from build123d import *

# Parameters (mm, degrees)
SKETCH1_R           = 46.355
BOSS_EXTRUDE1_DEPTH = 6.35
SKETCH2_R           = 20.955
BOSS_EXTRUDE2_DEPTH = 50.8
CUT_EXTRUDE1_REACH  = 59.15
SKETCH3_3_R         = 13.0175
CUT_EXTRUDE2_DEPTH  = 34.29
CUT_EXTRUDE3_REACH  = 48.355
SKETCH5_5_R         = 2.2479
CUT_EXTRUDE7_DEPTH  = 9.525
CIRPATTERN1_COUNT   = 4
CUT_EXTRUDE8_REACH  = 95.345
SKETCH6_R           = 2.60985
SKETCH6_4_R         = 4.7625
CUT_EXTRUDE9_DEPTH  = 32.72
CHAMFER1_SIZE       = 1


with BuildPart() as part:
    # Sketch1 → Boss-Extrude1 (new body)
    with BuildSketch(Plane(origin=(0, 0, 0), x_dir=(1, 0, 0), z_dir=(0, 1, 0))):
        Circle(SKETCH1_R)
    extrude(amount=BOSS_EXTRUDE1_DEPTH)

    # Sketch2 → Boss-Extrude2 (add)
    with BuildSketch(Plane(origin=(0, 6.35, 0), x_dir=(1, 0, 0), z_dir=(0, 1, 0))):
        Circle(SKETCH2_R)
    extrude(amount=BOSS_EXTRUDE2_DEPTH)

    # Sketch3 → Cut-Extrude1 (cut, up to next)
    with BuildSketch(Plane(origin=(0, 57.15, 0), x_dir=(1, 0, 0), z_dir=(0, 1, 0)), mode=Mode.PRIVATE) as cut_extrude1_sk1:
        with BuildLine():
            Line((-2.84, -1.921572533), (-2.84, 1.921572533))
            ThreePointArc((-2.84, 1.921572533), (3.429, 0), (-2.84, -1.921572533))
        make_face()
    cut_extrude1_tool1 = extrude(cut_extrude1_sk1.sketch, amount=-CUT_EXTRUDE1_REACH, mode=Mode.PRIVATE) & part.part
    add(cut_extrude1_tool1.solids().sort_by_distance((0.133614, 57.15, 0))[0], mode=Mode.SUBTRACT)

    # Sketch3_3 → Cut-Extrude2 (cut)
    with BuildSketch(Plane(origin=(0, 57.15, 0), x_dir=(1, 0, 0), z_dir=(0, 1, 0))):
        Circle(SKETCH3_3_R)
    extrude(amount=-CUT_EXTRUDE2_DEPTH, mode=Mode.SUBTRACT)

    # Sketch4 → Cut-Extrude3 (cut, up to next)
    with BuildSketch(Plane(origin=(0, 0, 0), x_dir=(0, 0, -1), z_dir=(1, 0, 0)), mode=Mode.PRIVATE) as cut_extrude3_sk1:
        with BuildLine():
            ThreePointArc((7.9375, 33.02), (0, 25.0825), (-7.9375, 33.02))
            Line((-7.9375, 33.02), (-7.9375, 38.1))
            ThreePointArc((-7.9375, 38.1), (0, 46.0375), (7.9375, 38.1))
            Line((7.9375, 38.1), (7.9375, 33.02))
        make_face()
    cut_extrude3_tool1 = extrude(cut_extrude3_sk1.sketch, amount=CUT_EXTRUDE3_REACH, mode=Mode.PRIVATE) & part.part
    add(cut_extrude3_tool1.solids().sort_by_distance((0, 35.56, 0))[0], mode=Mode.SUBTRACT)

    # Sketch5_5 → Cut-Extrude7 (cut)
    with BuildSketch(Plane.XZ.offset(-57.15)):
        with Locations((0, -16.98625)):
            Circle(SKETCH5_5_R)
    cut_extrude7 = extrude(amount=CUT_EXTRUDE7_DEPTH, mode=Mode.SUBTRACT)

    # CirPattern1: Cut-Extrude7 ×4 about axis
    cirpattern1_axis = Axis((0, 0, 0), (0, 1, 0))
    for i in range(1, CIRPATTERN1_COUNT):
        add(cut_extrude7.rotate(cirpattern1_axis, i * 360 / CIRPATTERN1_COUNT), mode=Mode.SUBTRACT)

    # Sketch6 → Cut-Extrude8 (cut, up to next)
    with BuildSketch(Plane(origin=(-46.99, 0, 0), x_dir=(0, 0, -1), z_dir=(1, 0, 0)), mode=Mode.PRIVATE) as cut_extrude8_sk1:
        with Locations((0, 7.62)):
            Circle(SKETCH6_R)
    cut_extrude8_tool1 = extrude(cut_extrude8_sk1.sketch, amount=CUT_EXTRUDE8_REACH, mode=Mode.PRIVATE) & part.part
    add(cut_extrude8_tool1.solids().sort_by_distance((-46.99, 7.62, 0))[0], mode=Mode.SUBTRACT)

    # Sketch6_4 → Cut-Extrude9 (cut)
    with BuildSketch(Plane(origin=(-46.99, 0, 0), x_dir=(0, 0, -1), z_dir=(1, 0, 0))):
        with Locations((0, 7.62)):
            Circle(SKETCH6_4_R)
    extrude(amount=CUT_EXTRUDE9_DEPTH, mode=Mode.SUBTRACT)

    # Chamfer1
    chamfer1_edges = [part.edges().sort_by_distance(p)[0] for p in [
        (-46.355, 0, 0),
        (2.297847054, 6.35, 46.298012095),
    ]]
    chamfer(chamfer1_edges, length=CHAMFER1_SIZE)


solid = part.part
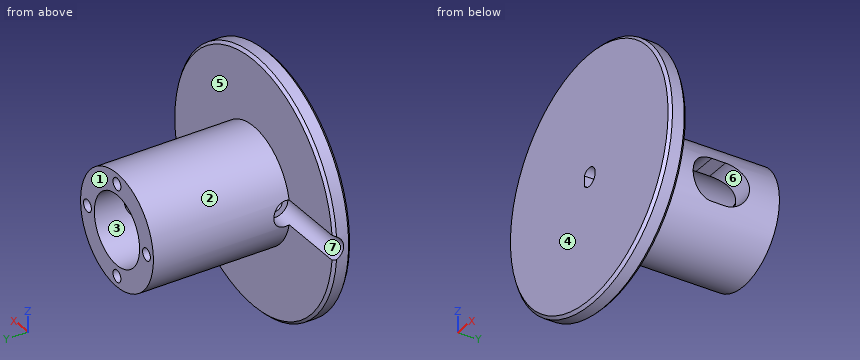
Model file for the job. Use its own axes, mm. Face numbers are marked on the shaded views. A direction names the side the tool comes from. Round coordinates to 2 decimals unless told otherwise and drop trailing zeros. Order: outer loops, then holes, each group sorted by start corner. A loop starts at its lowest first (then second) coordinate and runs counter-clockwise, first axis right, second up.
(1) Drill centre lines: line 1 (Z direction, x = 0, y = 55.25) (1 decimal); line 2 (X direction, y = 48, z = -1.5). Where is each one in solid material? Low to high.
(2) Band-saw the part on B-B (z = 0). Give the number of separate pieces and of enclosed holes in the cut face, then the cut area to 3 significant figures.
(3) Pin check, flat tips, straight feed: pin 1 (13 mm diameter, centred on x = 1, z = 6, fed in from +Y); pin 2 (3.5 mm diameter, centred on x = -1, z = 17.5, fed in from +Y); pin 3 (4 mm diameter, centred on y = 19, z = 0, fed in from +X) (3 decimals); pin 4 (1 mm diameter, centred on x = -19, y = 45.5, fed in from +Z). Stop position of each tip, or through.
(4) Band-saw the part on C-C (y = 19.5). List the corners of the cut face in (x, z) (3 decimals), then the cut area to 3 significant figures.
(5) Pull direction X, two halves, no side cores. Call the marked faces 1, 2 and 3: released by +X, released by -X, zero draft, split by the parting line, or undercut.
(6) Band-saw the part on D-D (y = 7.62). List the corners of the cut face in (x, z) (1 decimal).
(7) 3-axis set-ups, long thin cutter, end or side, ignore diameter. For the marked faces 4, 5, 6 and 7: which of +Z, -Z, +X, -X, +Y, -Y reach the whole face in a straight line?
Verdict:
1. line 1: z = -21 to -19.2, -14.7 to -13, 13 to 14.7, 19.2 to 21
1. line 2: x = -20.9 to -18.66, -15.31 to -12.93, 12.93 to 15.31, 18.66 to 20.9
2. separate pieces: 4
2. enclosed holes: 0
2. area: 1,220 mm2
3. pin 1: stops at y = 22.86
3. pin 2: stops at y = 57.15
3. pin 3: stops at x = 20.955
3. pin 4: stops at z = 9.84
4. outline: circle Ø41.91 at (0, 0); hole (-2.84, -1.922) arc R3.429 ccw (long way) to (-2.84, 1.922) - close
4. area: 1,340 mm2
5. face 1: zero draft
5. face 2: split by the parting line
5. face 3: undercut
6. outline: (-20.4, -4.8) arc R21 ccw (long way) to (-20.4, 4.8) - (-14.3, 4.8) - (-14.3, 2.6) - (-2.2, 2.6) arc R3.4 cw (long way) to (-2.2, -2.6) - (-14.3, -2.6) - (-14.3, -4.8) - close
7. face 4: +Z, -Z, +X, -X, -Y
7. face 5: +Y
7. face 6: +X
7. face 7: -X
